Design review of the part built by this model. Coordinates are the model's own, in mm. A direction names the side the tool comes from. Round coordinates to 2 decimals unless told otherwise and drop trailing zeros. Write each loop counter-clockwise with the first axis right and the second up, starting at its lowest first coordinate (ties: lowest second). Pieces come first, ordered by that corner, then holes. Notation, with made-up numbers: (20.5, 11) -> (29.5, 11) arc R27 ccw to (29.5, 36) -> close; hole circle Ø9 at (28, 77). An arc over 180 degrees is marked (long way). Write item = value, one per line. Start each with the question number.
Item 1: Add section C-C, the plane z = 7. State the section outline as (x, y) points, then the cut area to 3 significant figures.
Item 2: Add section B-B, the plane x = 0. State the section outline as (y, z) points, then the cut area to 3 significant figures.
Item 3: Add section D-D, the plane y = 4.5. State the section outline as (x, z) points.
Item 4: Machinability: for faces 4 (the cylindrical face through (1.87, -5.04, 4.44)), 5 (the flat face through (0, 3.05, 4)), which of the approach directions +Z, -Z, +X, -X, +Y, -Y give a long, thin tool a straight path to every point of the face, cutting with its end or side? Answer none if there is none.
Item 5: Add section A-A, the plane x = -2. State the section outline as (y, z) points, then the cut area to 3 significant figures.
Item 6: For pin 1 Ø1.6 at (x, y) = (-2, -6.03) entering from +Z; pin 2 Ø2.5 at (x, y) = (2, -6.03) entering from -Z, all flat-tipped, find the tip position at first contact; note any pin that passes through.
Item 7: Mouldability with a two-part tool opening along X and no side actions: class faces 1 (the cylindrical face through (5.377, -8.18, 4.563)), 2 (the cylindrical face through (-5.408, 8.149, 4.563)), 3 (the cylindrical face through (-2.13, -5.04, 4.44)) as released by +X, released by -X, zero draft, split by the parting line, or undercut.
Item 8: To check wall thickness, follow L1, parallel to Y at x = -2, z = 3.5; L2, parallel to X at y = 5.7, z = 4.5; L3, parallel to Y at x = 0, z = 4. State the ranges of each line that lie inside material, in increasing order.
from build123d import *

# Parameters (mm, degrees)
SKETCH1_W           = 11.957581354
SKETCH1_H           = 17.5
SKETCH1_R           = 1
BOSS_EXTRUDE1_DEPTH = 9
CUT_EXTRUDE1_START  = -2
SKETCH2_R           = 3.5
CUT_EXTRUDE1_DEPTH  = 3.7
FILLET1_R           = 2


with BuildPart() as part:
    # Sketch1 → Boss-Extrude1 (new body)
    with BuildSketch(Plane.XY):
        Rectangle(SKETCH1_W, SKETCH1_H)
        with Locations((-2, -6.032367874)):
            Circle(SKETCH1_R, mode=Mode.SUBTRACT)
        with Locations((2, -6.032367874)):
            Circle(SKETCH1_R, mode=Mode.SUBTRACT)
    extrude(amount=BOSS_EXTRUDE1_DEPTH)

    # Sketch2 → Cut-Extrude1 (cut)
    with BuildSketch(Plane(origin=(0, 8.75, 0), x_dir=(1, 0, 0), z_dir=(0, 1, 0)).offset(CUT_EXTRUDE1_START)):
        with Locations(Location((0, -4.5, 0), (0, 0, 270))):
            Circle(SKETCH2_R)
    extrude(amount=-CUT_EXTRUDE1_DEPTH, mode=Mode.SUBTRACT)

    # Fillet1
    fillet1_edges = [part.edges().sort_by_distance(p)[0] for p in [
        (5.978790677, -8.75, 4.5),
        (-5.978790677, -8.75, 4.5),
        (-5.978790677, 8.75, 4.5),
        (5.978790677, 8.75, 4.5),
    ]]
    fillet(fillet1_edges, radius=FILLET1_R)


solid = part.part
Result set:
q1.outline = (-5.98, -6.75) arc R2 ccw to (-3.98, -8.75) -> (3.98, -8.75) arc R2 ccw to (5.98, -6.75) -> (5.98, 6.75) arc R2 ccw to (3.98, 8.75) -> (-3.98, 8.75) arc R2 ccw to (-5.98, 6.75) -> close; hole circle Ø2 at (-2, -6.03); hole (-2.45, 3.05) -> (2.45, 3.05) -> (2.45, 6.75) -> (-2.45, 6.75) -> close; hole circle Ø2 at (2, -6.03)
q1.area = 181 mm²
q2.outline = (-8.75, 0) -> (8.75, 0) -> (8.75, 9) -> (-8.75, 9) -> close; hole (3.05, 1) -> (6.75, 1) -> (6.75, 8) -> (3.05, 8) -> close
q2.area = 132 mm²
q3.outline = (-5.98, 0) -> (5.98, 0) -> (5.98, 9) -> (-5.98, 9) -> close; hole circle Ø7 at (0, 4.5)
q4.face_4 = +Z, -Z
q4.face_5 = none
q5.outline = (-8.75, 0) -> (-7.03, 0) -> (-7.03, 9) -> (-8.75, 9) -> close; (-5.03, 0) -> (8.75, 0) -> (8.75, 9) -> (-5.03, 9) -> close; hole (3.05, 1.63) -> (6.75, 1.63) -> (6.75, 7.37) -> (3.05, 7.37) -> close
q5.area = 118 mm²
q6.pin_1 = through
q6.pin_2 = 0
q7.face_1 = released by +X
q7.face_2 = released by -X
q7.face_3 = undercut
q8.L1 = -8.75 to -7.03, -5.03 to 3.05, 6.75 to 8.75
q8.L2 = -5.98 to -3.5, 3.5 to 5.98
q8.L3 = -8.75 to 3.05, 6.75 to 8.75
